Design review of the part built by this model. Coordinates are the model's own, in mm. Face numbers are marked on the shaded views. Coordinates: 2 decimals unless noted, no trailing zeros. Write each loop counter-clockwise with the first axis right and the second up, starting at its lowest first coordinate (ties: lowest second). Pieces come first, ordered by that corner, then holes.
Q1. Take a section at C-C (x = 13). Give the boundary of the cut face in (y, z).
Q2. Insertion check: pin 1 (1 mm diameter, centred on x = 10.5, y = 3.5, fed in from +Z); pin 2 (1.4 mm diameter, centred on x = 0.5, y = -0.5, fed in from -Z); pin 3 (2 mm diameter, centred on x = 44.5, y = 3, fed in from -Z). Each pin has a flat end and moves straight along its axis. Give the tip position at first contact, or say it passes through.
Q3. Mouldability with a two-part tool opening along Z and no side actions: class the marked faces 1 and 2 as pulls with the +Z half, pulls with the -Z half, needs draft (parallel to the pull), parting line crosses it, or undercut.
Q4. Take a section at B-B (x = 83). Give the boundary of the cut face in (y, z), and give its area (3 significant figures).
Q5. For probe 1 along X at (y, z) = (2.15, -28); probe 2 along Z at (x, y) = (13, 0.95); probe 3 along X at (y, z) = (2.7, -30), list the stretches that pass through material, from the lowest coordinate up.
Q6. Take a section at A-A (x = 40). Give the boundary of the cut face in (y, z).
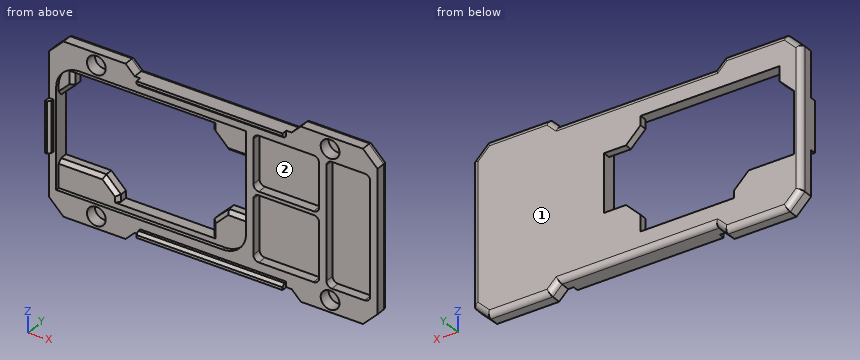
```python
from build123d import *

# Parameters (mm, degrees)
SKETCH1_W           = 90
SKETCH1_H           = 47
BOSS_EXTRUDE1_DEPTH = 4
CUT_EXTRUDE1_START  = -4
CUT_EXTRUDE1_DEPTH  = 106.612007165
FILLET1_R           = 6.4
CUT_EXTRUDE3_START  = -4
SKETCH4_R           = 2.57
CUT_EXTRUDE3_DEPTH  = 3.2
SKETCH5_W           = 20
SKETCH5_H           = 4
CUT_EXTRUDE4_DEPTH  = 21.1
CHAMFER1_SIZE       = 4
BOSS_EXTRUDE2_DEPTH = 3
CHAMFER2_SIZE       = 4
CHAMFER3_SIZE       = 4
SKETCH7_W           = 12
SKETCH7_H           = 34
CUT_EXTRUDE5_DEPTH  = 2.5
FILLET2_R           = 1.5
CHAMFER4_SIZE       = 1
BOSS_EXTRUDE3_DEPTH = 5.5
CUT_EXTRUDE6_DEPTH  = 1.5
FILLET3_R           = 1.5
BOSS_EXTRUDE4_DEPTH = 1.5
CHAMFER6_SIZE       = 0.75


with BuildPart() as part:
    # Sketch1 → Boss-Extrude1 (new body)
    with BuildSketch(Plane(origin=(0, 0, 0), x_dir=(1, 0, 0), z_dir=(0, 1, 0))):
        with Locations((45, 23.5)):
            Rectangle(SKETCH1_W, SKETCH1_H)
    extrude(amount=BOSS_EXTRUDE1_DEPTH)

    # Sketch2 → Cut-Extrude1 (cut, through all)
    with BuildSketch(Plane(origin=(0, 4, 0), x_dir=(1, 0, 0), z_dir=(0, 1, 0)).offset(CUT_EXTRUDE1_START)):
        Polygon((2, 23.5), (2, 40.5), (54, 40.5), (54, 6.5), (2, 6.5), align=None)
    extrude(amount=CUT_EXTRUDE1_DEPTH, mode=Mode.SUBTRACT)

    # Fillet1
    fillet1_edges = [part.edges().sort_by_distance(p)[0] for p in [
        (54, 2, -40.5),
        (2, 2, -6.5),
    ]]
    fillet(fillet1_edges, radius=FILLET1_R)

    # Sketch4 → Cut-Extrude3 (cut)
    with BuildSketch(Plane(origin=(0, 4, 0), x_dir=(1, 0, 0), z_dir=(0, 1, 0)).offset(CUT_EXTRUDE3_START)):
        with Locations(Location((13, 43.75, 0), (0, 0, 90))):
            Circle(SKETCH4_R)
        with Locations(Location((13, 3.25, 0), (0, 0, 90))):
            Circle(SKETCH4_R)
        with Locations(Location((77, 3.25, 0), (0, 0, 90))):
            Circle(SKETCH4_R)
        with Locations(Location((77, 43.75, 0), (0, 0, 90))):
            Circle(SKETCH4_R)
    extrude(amount=CUT_EXTRUDE3_DEPTH, mode=Mode.SUBTRACT)

    # Sketch5 → Cut-Extrude4 (cut)
    with BuildSketch(Plane(origin=(0, 4, 0), x_dir=(1, 0, 0), z_dir=(0, 1, 0))):
        with Locations((35, 2)):
            Rectangle(SKETCH5_W, SKETCH5_H)
        with Locations((55, 2)):
            Rectangle(SKETCH5_W, SKETCH5_H)
        with Locations((35, 45)):
            Rectangle(SKETCH5_W, SKETCH5_H)
        with Locations((55, 45)):
            Rectangle(SKETCH5_W, SKETCH5_H)
    extrude(amount=-CUT_EXTRUDE4_DEPTH, mode=Mode.SUBTRACT)

    # Chamfer1
    chamfer1_edges = [part.edges().sort_by_distance(p)[0] for p in [
        (90, 2, 0),
        (90, 2, -47),
        (0, 2, -47),
        (0, 2, 0),
        (25, 2, -47),
        (65, 2, -47),
        (65, 2, 0),
        (25, 2, 0),
    ]]
    chamfer(chamfer1_edges, length=CHAMFER1_SIZE - 0.0001)  # a hair under: the kernel refuses the full size

    # Sketch6 → Boss-Extrude2 (add)
    with BuildSketch(Plane(origin=(0, 4, 0), x_dir=(1, 0, 0), z_dir=(0, 1, 0))):
        Polygon((54, 6.5), (54, 14.5), (44, 14.5), (44, 8), (6, 8), (6, 16), (2, 16), (2, 6.5), (42, 6.5), align=None)
        Polygon((47.6, 40.5), (54, 40.5), (54, 30.5), (44, 30.5), (44, 39), (18.412776199, 39), (18.412776199, 33), (2, 33), (2, 40.5), align=None)
    extrude(amount=-BOSS_EXTRUDE2_DEPTH)

    # Chamfer2
    chamfer2_edges = [part.edges().sort_by_distance(p)[0] for p in [
        (44, 2.5, -14.5),
        (44, 2.5, -30.5),
        (18.412776199, 2.5, -33),
    ]]
    chamfer(chamfer2_edges, length=CHAMFER2_SIZE)

    # Chamfer3
    chamfer3_edges = [part.edges().sort_by_distance(p)[0] for p in [
        (6, 2.5, -16),
    ]]
    chamfer(chamfer3_edges, length=CHAMFER3_SIZE - 0.0001)  # a hair under: the kernel refuses the full size

    # Sketch7 → Cut-Extrude5 (cut)
    with BuildSketch(Plane.XZ):
        Polygon((65, -22.5), (56, -22.5), (56, -40.5), (74, -40.5), (74, -22.5), align=None)
        Polygon((56, -6.5), (74, -6.5), (74, -21.5), (65, -21.5), (56, -21.5), align=None)
        with Locations((82, -23.5)):
            Rectangle(SKETCH7_W, SKETCH7_H)
    extrude(amount=-CUT_EXTRUDE5_DEPTH, mode=Mode.SUBTRACT)

    # Fillet2
    fillet2_edges = [part.edges().sort_by_distance(p)[0] for p in [
        (76, 1.25, -6.5),
        (88, 1.25, -6.5),
        (88, 1.25, -40.5),
        (76, 1.25, -40.5),
        (56, 1.25, -21.5),
        (56, 1.25, -6.5),
        (74, 1.25, -6.5),
        (74, 1.25, -21.5),
        (74, 1.25, -22.5),
        (74, 1.25, -40.5),
        (56, 1.25, -40.5),
        (56, 1.25, -22.5),
    ]]
    fillet(fillet2_edges, radius=FILLET2_R)

    # Chamfer4
    chamfer4_edges = [part.edges().sort_by_distance(p)[0] for p in [
        (6, 1, -10.00005),
        (51, 1, -14.5),
        (44, 1, -36.75),
        (8.206388099, 1, -33),
        (18.412776199, 1, -38),
        (51, 1, -30.5),
        (46, 1, -32.5),
        (16.412776199, 1, -35),
        (44, 1, -9.25),
        (46, 1, -12.5),
        (4.00005, 1, -14.00005),
    ]]
    chamfer(chamfer4_edges, length=CHAMFER4_SIZE)

    # Sketch8 → Boss-Extrude3 (add)
    with BuildSketch(Plane(origin=(0, 4, 0), x_dir=(1, 0, 0), z_dir=(0, 1, 0))):
        Polygon((65, 4), (45, 4), (45, 2.5), (66.5, 2.5), align=None)
        Polygon((45, 2.5), (45, 4), (25, 4), (23.5, 2.5), align=None)
        Polygon((66.5, 44.5), (45, 44.5), (45, 43), (65, 43), align=None)
        Polygon((45, 44.5), (23.5, 44.5), (25, 43), (45, 43), align=None)
    extrude(amount=-BOSS_EXTRUDE3_DEPTH)

    # Sketch10 → Cut-Extrude6 (cut)
    with BuildSketch(Plane(origin=(0, -1.5, 0), x_dir=(-1, 0, 0), z_dir=(0, -1, 0))):
        Polygon((-25, 4), (-25, 2.5), (-23.5, 2.5), align=None)
        Polygon((-65, 4), (-65, 2.5), (-66.5, 2.5), align=None)
        Polygon((-65, 43), (-65, 44.5), (-66.5, 44.5), align=None)
        Polygon((-25, 43), (-25, 44.5), (-23.5, 44.5), align=None)
    extrude(amount=-CUT_EXTRUDE6_DEPTH, mode=Mode.SUBTRACT)

    # Fillet3
    fillet3_edges = [part.edges().sort_by_distance(p)[0] for p in [
        (77.5, 4, 0),
        (90, 4, -23.5),
        (77.5, 4, -47),
        (12.5, 4, -47),
        (0, 4, -23.5),
        (12.5, 4, 0),
        (1.99995, 4, -1.99995),
        (1.99995, 4, -45.00005),
        (88.00005, 4, -45.00005),
        (88.00005, 4, -1.99995),
        (22.2501, 4, -1.25),
        (67.7499, 4, -45.75),
        (67.7499, 4, -1.25),
        (45, 4, -2.5),
        (22.2501, 4, -45.75),
        (45, 4, -44.5),
    ]]
    fillet(fillet3_edges, radius=FILLET3_R)

    # Sketch11 → Boss-Extrude4 (add)
    with BuildSketch(Plane.XZ):
        Polygon((0, -23.5), (0, -16.5), (1.25, -16.5), (1.25, -30.5), (0, -30.5), align=None)
    extrude(amount=BOSS_EXTRUDE4_DEPTH)

    # Chamfer6
    chamfer6_edges = [part.edges().sort_by_distance(p)[0] for p in [
        (45, -1.5, -4),
        (45, -1.5, -43),
        (1.25, -1.5, -23.5),
    ]]
    chamfer(chamfer6_edges, length=CHAMFER6_SIZE)


solid = part.part
```
Response:
1. outline: (0, -47) - (2.5, -47) arc R1.5 ccw to (4, -45.5) - (4, -33) - (2, -33) - (1, -34) - (1, -40.5) - (0, -40.5) - (0, -41.18) - (3.2, -41.18) - (3.2, -46.32) - (0, -46.32) - close; (0, -6.5) - (1, -6.5) - (1, -8) - (4, -8) - (4, -1.5) arc R1.5 ccw to (2.5, 0) - (0, 0) - (0, -0.68) - (3.2, -0.68) - (3.2, -5.82) - (0, -5.82) - close
2. pin 1: stops at z = -0.09
2. pin 2: stops at z = -43.99
2. pin 3: stops at z = -44.5
3. face 1: needs draft
3. face 2: undercut
4. outline: (0, -47) - (2.5, -47) arc R1.5 ccw to (4, -45.5) - (4, -1.5) arc R1.5 ccw to (2.5, 0) - (0, 0) - (0, -6.5) - (2.5, -6.5) - (2.5, -40.5) - (0, -40.5) - close
4. area: 102 mm2
5. probe 1: x = 0 to 2, 54 to 56, 74 to 76, 88 to 90
5. probe 2: z = -47 to -46.32, -41.18 to -40.5, -6.5 to -5.82, -0.68 to 0
5. probe 3: x = 0.01 to 2, 54 to 89.99
6. outline: (-1.5, -44.5) - (2.5, -44.5) arc R1.5 ccw to (4, -43) - (4, -39) - (1, -39) - (1, -40.5) - (0, -40.5) - (0, -43) - (-0.75, -43) - (-1.5, -43.75) - close; (-1.5, -3.25) - (-0.75, -4) - (0, -4) - (0, -6.5) - (1, -6.5) - (1, -8) - (4, -8) - (4, -4) arc R1.5 ccw to (2.5, -2.5) - (-1.5, -2.5) - close
